```python
from build123d import *

# Parameters (mm, degrees)
F0_W     = 19.05
F0_H     = 19.05
F0_W_2   = 15.9766
F0_H_2   = 15.9766
F1_DEPTH = 69.85
F2_R     = 1.86055
F3_DEPTH = 19.05


with BuildPart() as f1:
    # F0 (on Front) → F1 (new body)
    with BuildSketch(Plane.XZ):
        Rectangle(F0_W, F0_H)
        Rectangle(F0_W_2, F0_H_2, mode=Mode.SUBTRACT)
    extrude(amount=F1_DEPTH)

    # F2 (on face) → F3 (cut, through all)
    with BuildSketch(Plane.XY.offset(9.525)):
        with Locations((0, -26.925)):
            Circle(F2_R)
        with Locations((0, -42.925)):
            Circle(F2_R)
    extrude(amount=-F3_DEPTH, mode=Mode.SUBTRACT)


solid = f1.part
```
Input: part model. Units: mm. Frame: model coordinates. A direction names the side the tool comes from. Give positions to 0.01 mm unless a question says otherwise; leave off trailing zeros. Order: outer loops, then holes, each group sorted by start corner. A loop starts at its lowest first (then second) coordinate and runs counter-clockwise, first axis right, second up.
1. Cut plane D-D (y = -21). Return loops of the section in (x, z) (3 decimals).
Computed:
outline: (-9.525, -9.525) - (9.525, -9.525) - (9.525, 9.525) - (-9.525, 9.525) - close; hole (-7.988, -7.988) - (7.988, -7.988) - (7.988, 7.988) - (-7.988, 7.988) - close
2. Cut plane B-B (x = 0). Return loops of the section in (y, z) (3 decimals).
Computed:
outline: (-69.85, -9.525) - (-44.786, -9.525) - (-44.786, -7.988) - (-69.85, -7.988) - close; (-69.85, 7.988) - (-44.786, 7.988) - (-44.786, 9.525) - (-69.85, 9.525) - close; (-41.064, -9.525) - (-28.786, -9.525) - (-28.786, -7.988) - (-41.064, -7.988) - close; (-41.064, 7.988) - (-28.786, 7.988) - (-28.786, 9.525) - (-41.064, 9.525) - close; (-25.064, -9.525) - (0, -9.525) - (0, -7.988) - (-25.064, -7.988) - close; (-25.064, 7.988) - (0, 7.988) - (0, 9.525) - (-25.064, 9.525) - close
3. Set-up query: faces 1 (the face through (-0.4, -44.74, 8.77)), 2 (the face through (0, -34, -7.988)). Return all of +Z, -Z, +X, -X, +Y, -Y with unobstructed straight access to the full face (end or side cutting, diameter ignored); none if empty.
Computed:
face 1: +Z, -Z
face 2: +Y, -Y
4. Line query: probe 1 along Y at (x, z) = (0, -8.8); probe 2 along Z at (x, y) = (-1, -12.5) (3 decimals). Output: solid intervals per line, ascending.
Computed:
probe 1: y = -69.85 to -44.79, -41.06 to -28.79, -25.06 to 0
probe 2: z = -9.525 to -7.988, 7.988 to 9.525
5. Cut plane A-A (z = 7). Return loops of the section in (x, y) (3 decimals), and give its area (3 significant figures).
Computed:
outline: (-9.525, -69.85) - (-7.988, -69.85) - (-7.988, 0) - (-9.525, 0) - close; (7.988, -69.85) - (9.525, -69.85) - (9.525, 0) - (7.988, 0) - close
area: 215 mm2
6. Cut plane C-C (x = -5.5). Return loops of the section in (y, z) (3 decimals).
Computed:
outline: (-69.85, -9.525) - (0, -9.525) - (0, -7.988) - (-69.85, -7.988) - close; (-69.85, 7.988) - (0, 7.988) - (0, 9.525) - (-69.85, 9.525) - close
7. Draft query along Y for faces 3 (the face through (-9, -69.85, 0)), 4 (the face through (0, -34, 7.988)), 5 (the face through (-9, 0, 0)), 6 (the face through (-0.24, -25.08, 8.77)). Return one class per face: released by +Y, released by -Y, zero draft, split by the parting line, or undercut.
Computed:
face 3: released by -Y
face 4: zero draft
face 5: released by +Y
face 6: undercut
